Check sheet for the modelled part. Datum: model origin and axes. Units: mm. A direction names the side the tool comes from. Round coordinates to 2 decimals unless told otherwise and drop trailing zeros. Loops run counter-clockwise (first coordinate to the right, second up) from the corner with the lowest first, then second, coordinate; pieces in that order, holes last. Notation, with made-up numbers: (31.25, 34) - (59.25, 34) arc R20 ccw to (59.25, 54) - close; hole circle Ø2 at (88.5, 65). An arc over 180 degrees is marked (long way). Put each result on its own line as item: value. Start each with the question number.
Item 1: Gauge pin test, flat ends, axial feed: pin 1 Ø1.5 at (x, y) = (4, 2) entering from -Z; pin 2 Ø2 at (x, z) = (2, 1) entering from -Y; pin 3 Ø1.3 at (x, z) = (3, 7) entering from -Y. Record the tip position at first contact, or that the pin passes through.
Item 2: Section check A-A, the plane y = 10. Record the cut outline in (x, z), and give its area (3 significant figures).
Item 3: Section check C-C, the plane z = 2. Record the cut outline in (x, y).
Item 4: Material ranges on line 1 along Z through (x, y) = (3, 1.6); line 2 along X through (y, z) = (2.6, 7); line 3 along Y through (x, z) = (3, 2.5), recorded low to high.
Item 5: Tool access check on faces 4 (the cylindrical face through (3.104, 2.535, 7.793)), 5 (the flat face through (3, 6.003, 9)), 6 (the flat face through (0.5, 3, 1)). Record the directions out of +Z, -Z, +X, -X, +Y, -Y that give a thin tool (end or side, any length) a straight path to the whole face; none if there is none.
Item 6: Draft check along X on faces 1 (the flat face through (5.5, 3, 1)), 2 (the flat face through (3, 7, 8)), 3 (the flat face through (6, 7, 5)). Enter one of: pulls with the +X half, pulls with the -X half, needs draft (parallel to the pull), parting line crosses it, or undercut.
Item 7: Section check D-D, the plane x = 4.7. Record the cut outline in (y, z), and give its area (3 significant figures).
Item 8: Section check B-B, the plane y = 3.5. Record the cut outline in (x, z).
from build123d import *

# Parameters (mm, degrees)
SKETCH_1_R             = 2.5
EXTRUDE_1_DEPTH        = 8
SKETCH_5_W             = 6
SKETCH_5_H             = 6.003393665
EXTRUDE_4_DEPTH        = 2
SKETCH_6_W             = 5
SKETCH_6_H             = 6
EXTRUDE_5_DEPTH        = 5
HOLE_WIZARD_M2_1_D     = 1.6
HOLE_WIZARD_M2_1_DEPTH = 5
HOLE_WIZARD_M2_1_TIP   = 0.480688495


with BuildPart() as part:
    # 스케치1 → 돌출1 (new body)
    with BuildSketch(Plane.XY):
        Polygon((0, 0), (0.5, 0), (0.5, 6), (5.5, 6), (5.5, 0), (6, 0), (6, 13.5), (0, 13.5), align=None)
        with Locations((3, 10)):
            Circle(SKETCH_1_R, mode=Mode.SUBTRACT)
    extrude(amount=EXTRUDE_1_DEPTH)

    # 스케치5 → 돌출4 (add)
    with BuildSketch(Plane.XY.offset(8)):
        with Locations((3, 3.001696832)):
            Rectangle(SKETCH_5_W, SKETCH_5_H)
    extrude(amount=EXTRUDE_4_DEPTH)

    # 스케치6 → 돌출5 (add)
    with BuildSketch(Plane(origin=(0, 0, 8), x_dir=(-1, 0, 0), z_dir=(0, 0, -1))):
        with Locations((-3, 3)):
            Rectangle(SKETCH_6_W, SKETCH_6_H)
    extrude(amount=EXTRUDE_5_DEPTH)

    # M2 탭을 위한 탭 드릴1
    with Locations(Plane.XZ):
        with Locations((3, 7)):
            Hole(HOLE_WIZARD_M2_1_D / 2, depth=HOLE_WIZARD_M2_1_DEPTH)
            with Locations((0, 0, -(HOLE_WIZARD_M2_1_DEPTH + HOLE_WIZARD_M2_1_TIP / 2))):  # 118° drill point
                Cone(0, HOLE_WIZARD_M2_1_D / 2, HOLE_WIZARD_M2_1_TIP, mode=Mode.SUBTRACT)


solid = part.part
Check result:
1. pin 1: z = 3
1. pin 2: y = 6
1. pin 3: y = 5.09
2. outline: (0, 0) - (0.5, 0) - (0.5, 8) - (0, 8) - close; (5.5, 0) - (6, 0) - (6, 8) - (5.5, 8) - close
2. area: 8.00 mm²
3. outline: (0, 0) - (0.5, 0) - (0.5, 6) - (5.5, 6) - (5.5, 0) - (6, 0) - (6, 13.5) - (0, 13.5) - close; hole circle Ø5 at (3, 10)
4. line 1: 3 to 6.2, 7.8 to 10
4. line 2: 0 to 2.2, 3.8 to 6
4. line 3: 6 to 7.5, 12.5 to 13.5
5. face 4: -Y
5. face 5: +Z, +X, -X, +Y
5. face 6: -Z, -Y
6. face 1: undercut
6. face 2: needs draft
6. face 3: pulls with the +X half
7. outline: (0, 3) - (6, 3) - (6, 0) - (8.17, 0) - (8.17, 8) - (6, 8) - (6, 10) - (0, 10) - close; (11.83, 0) - (13.5, 0) - (13.5, 8) - (11.83, 8) - close
7. area: 72.7 mm²
8. outline: (0, 0) - (0.5, 0) - (0.5, 3) - (5.5, 3) - (5.5, 0) - (6, 0) - (6, 10) - (0, 10) - close; hole circle Ø1.6 at (3, 7)
